```python
from build123d import *

# Parameters (mm, degrees)
F1_DEPTH  = 1.5875
F2_W      = 10.16
F2_H      = 3.175
F3_DEPTH  = 33.02
F5_DEPTH  = 1.5875
F7_DEPTH  = 4.1275
F8_R      = 1.5875
F9_DEPTH  = 50.8
F10_R     = 1.5875
F11_DEPTH = 50.8


with BuildPart() as f1:
    # F0 (on Front) → F1 (new body)
    with BuildSketch(Plane.XZ):
        Polygon((-11.134821, 14.270418), (-16.214821, 9.190418), (-16.214821, -16.209582), (-6.054821, -16.209582), (-6.054821, 14.270418), align=None)
    extrude(amount=F1_DEPTH)

    # F2 (on face) → F3 (join)
    with BuildSketch(Plane.XZ.offset(1.5875)):
        with Locations((-11.134821, 2.522918)):
            Rectangle(F2_W, F2_H)
    extrude(amount=F3_DEPTH)

    # F4 (on face) → F5 (join)
    with BuildSketch(Plane.XZ.offset(34.6075)):
        Polygon((-16.214821, 9.190418), (-16.214821, 4.110418), (-16.214821, 0.935418), (-16.214821, -16.209582), (-6.054821, -16.209582), (-6.054821, 0.935418), (-6.054821, 4.110418), (-6.054821, 14.270418), (-11.134821, 14.270418), align=None)
    extrude(amount=F5_DEPTH)

    # F6 (on face) → F7 (join)
    with BuildSketch(Plane(origin=(0, 0, 0), x_dir=(-1, 0, 0), z_dir=(0, 1, 0))):
        Polygon((6.054821, -16.209582), (16.214821, -16.209582), (16.214821, 9.190418), (11.134821, 14.270418), (6.054821, 14.270418), align=None)
    extrude(amount=F7_DEPTH)

    # F8 (on face) → F9 (cut)
    with BuildSketch(Plane.XZ.offset(36.195)):
        with Locations((-11.134821, -10.812082)):
            Circle(F8_R)
    extrude(amount=-F9_DEPTH, mode=Mode.SUBTRACT)

    # F10 (on face) → F11 (cut)
    with BuildSketch(Plane.XZ.offset(36.195)):
        with Locations((-11.134821, 9.190418)):
            Circle(F10_R)
    extrude(amount=-F11_DEPTH, mode=Mode.SUBTRACT)


solid = f1.part
```
Input: part model. Units: mm. Frame: model coordinates. A direction names the side the tool comes from. Coordinates: 2 decimals unless noted, no trailing zeros. Write each loop counter-clockwise with the first axis right and the second up, starting at its lowest first coordinate (ties: lowest second). Pieces come first, ordered by that corner, then holes.
1) Section A-A on z = -13. Output: boundary loops of the cut face in (x, y) (1 decimal), and give its area (3 significant figures).
2) Set-up query: faces 1 (the flat face through (-11, -18, 4.11)), 2 (the flat face through (-13.639, -35.39, 11.766)), 3 (the flat face through (-11, -34.608, -8)). Return all of +Z, -Z, +X, -X, +Y, -Y with unobstructed straight access to the full face (end or side cutting, diameter ignored); none if empty.
3) Section D-D on x = -7. Output: boundary loops of the cut face in (y, z) (1 decimal), and give its area (3 significant figures).
4) Section B-B on x = -11.75. Output: boundary loops of the cut face in (y, z) (1 decimal).
5) Material intervals for line 1 along Y through (x, z) = (-8.25, -1.5) (1 decimal); line 2 along Z through (x, y) = (-7.5, -17.5), sorted ascending.
6) Section C-C on y = 0.5. Output: boundary loops of the cut face in (x, z) (1 decimal).
7) Mould query, pull axis Z, two halves, no side actions, for faces 4 (the flat face through (-11, 1, -16.21)), 5 (the flat face through (-16.215, -17.6, 1.1)), 6 (the flat face through (-9, 1, 14.27)), 7 (the cylindrical face through (-12.395, -35.412, -11.778)). Classes: pulls with the +Z half, pulls with the -Z half, needs draft (parallel to the pull), parting line crosses it, or undercut.
8) Pin query (flat end, axial travel): pin 1 Ø4 at (x, y) = (-8, -28.5) entering from -Z; pin 2 Ø5 at (x, z) = (-11.13, -10.81) entering from -Y (3 decimals); pin 3 Ø6 at (x, y) = (-10.5, -16.5) entering from +Z. Return the tip coordinate at first contact, or that it passes through.
Check result:
1. outline: (-16.2, -36.2) - (-6.1, -36.2) - (-6.1, -34.6) - (-16.2, -34.6) - close; (-16.2, -1.6) - (-6.1, -1.6) - (-6.1, 4.1) - (-16.2, 4.1) - close
1. area: 74.2 mm2
2. face 1: +Z, +X, -X
2. face 2: +Z, -X, +Y, -Y
2. face 3: -Z, +X, -X
3. outline: (-36.2, -16.2) - (-34.6, -16.2) - (-34.6, 0.9) - (-1.6, 0.9) - (-1.6, -16.2) - (4.1, -16.2) - (4.1, 14.3) - (-1.6, 14.3) - (-1.6, 4.1) - (-34.6, 4.1) - (-34.6, 14.3) - (-36.2, 14.3) - close
3. area: 327 mm2
4. outline: (-36.2, -16.2) - (-34.6, -16.2) - (-34.6, -12.3) - (-36.2, -12.3) - close; (-36.2, -9.3) - (-34.6, -9.3) - (-34.6, 0.9) - (-1.6, 0.9) - (-1.6, -9.3) - (4.1, -9.3) - (4.1, 7.7) - (-1.6, 7.7) - (-1.6, 4.1) - (-34.6, 4.1) - (-34.6, 7.7) - (-36.2, 7.7) - close; (-36.2, 10.7) - (-34.6, 10.7) - (-34.6, 13.7) - (-36.2, 13.7) - close; (-1.6, -16.2) - (4.1, -16.2) - (4.1, -12.3) - (-1.6, -12.3) - close; (-1.6, 10.7) - (4.1, 10.7) - (4.1, 13.7) - (-1.6, 13.7) - close
5. line 1: y = -36.2 to -34.6, -1.6 to 4.1
5. line 2: z = 0.94 to 4.11
6. outline: (-16.2, -16.2) - (-6.1, -16.2) - (-6.1, 14.3) - (-11.1, 14.3) - (-16.2, 9.2) - close; hole circle Ø3.2 at (-11.1, -10.8); hole circle Ø3.2 at (-11.1, 9.2)
7. face 4: pulls with the -Z half
7. face 5: needs draft
7. face 6: pulls with the +Z half
7. face 7: undercut
8. pin 1: stops at z = 0.94
8. pin 2: stops at y = -36.195
8. pin 3: stops at z = 4.11
